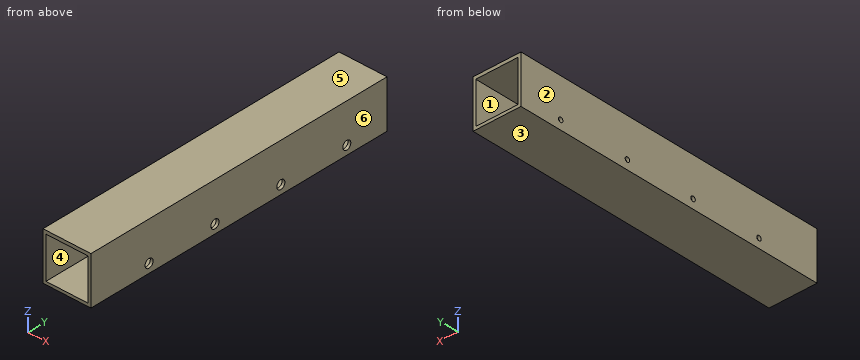
```python
from build123d import *

# Parameters (mm, degrees)
F0_W     = 50.8
F0_H     = 50.8
F0_W_2   = 44.7234460877
F0_H_2   = 44.0774458626
F1_DEPTH = 168.275
F3_D     = 9.144
F3_DEPTH = 25.4
F3_TIP   = 2.7471347502
F5_D     = 5.08
F5_DEPTH = 25.4
F5_TIP   = 1.5261859723


with BuildPart() as f1:
    # F0 (on Front) → F1 (new body, symmetric)
    with BuildSketch(Plane.XZ):
        with Locations((0.9841322899, 3.6690509832)):
            Rectangle(F0_W, F0_H)
        with Locations((1.1056640122, 3.467582593)):
            Rectangle(F0_W_2, F0_H_2, mode=Mode.SUBTRACT)
    extrude(amount=F1_DEPTH, both=True)

    # F3
    with Locations(Plane.YZ.offset(26.3841322899)):
        with Locations((-102.235, -12.3329490168), (-27.305, -12.3329490168), (47.625, -12.3329490168), (122.555, -12.3329490168)):
            Hole(F3_D / 2, depth=F3_DEPTH)
            with Locations((0, 0, -(F3_DEPTH + F3_TIP / 2))):  # 118° drill point
                Cone(0, F3_D / 2, F3_TIP, mode=Mode.SUBTRACT)

    # F5
    with Locations(Plane(origin=(-24.4158677101, 0, 0), x_dir=(0, -1, 0), z_dir=(-1, 0, 0))):
        with Locations((-123.0434924364, -12.0630878955), (-47.2589172423, -12.0630878955), (27.3903068155, -12.0630878955), (102.3233607411, -12.0630878955)):
            Hole(F5_D / 2, depth=F5_DEPTH)
            with Locations((0, 0, -(F5_DEPTH + F5_TIP / 2))):  # 118° drill point
                Cone(0, F5_D / 2, F5_TIP, mode=Mode.SUBTRACT)


solid = f1.part
```
Build history of the part. All positions in model axes, mm. Face numbers are marked on the shaded views. A direction names the side the tool comes from. Round coordinates to 2 decimals unless told otherwise and drop trailing zeros. Write each loop counter-clockwise with the first axis right and the second up, starting at its lowest first coordinate (ties: lowest second). Pieces come first, ordered by that corner, then holes.
1) Band-saw the part on B-B, the plane x = 6.5. List the corners of the cut face in (y, z) (3 decimals), and give its area (3 significant figures).
2) 3-axis set-ups, long thin cutter, end or side, ignore diameter. For the marked faces 1 and 2: which of +Z, -Z, +X, -X, +Y, -Y reach the whole face in a straight line?
3) Band-saw the part on C-C, the plane y = 6.5. List the corners of the cut face in (x, z).
4) Drill centre lines: probe 1 along Z at (x, y) = (-11.5, 6.5); probe 2 along X at (y, z) = (113, -2.5). Where is each one in solid material? Low to high.
5) Mould opens along Z. For the marked faces 3, 4, 5 and 6 say: +Z half, -Z half, draft (parallel to the pull), parting line (faces both ways), or undercut.
6) Pin check, flat tips, straight feed: pin 1 (4 mm diameter, centred on y = -102.32, z = -12.06, fed in from +X); pin 2 (7.5 mm diameter, centred on y = -27.3, z = -12.33, fed in from +X). Stop position of each tip, or through.
7) Band-saw the part on A-A, the plane z = 3. List the corners of the cut face in (x, y) (3 decimals), and give its area (3 significant figures).
Ans:
1. outline: (-168.275, -21.731) - (168.275, -21.731) - (168.275, -18.571) - (-168.275, -18.571) - close; (-168.275, 25.506) - (168.275, 25.506) - (168.275, 29.069) - (-168.275, 29.069) - close
1. area: 2,260 mm2
2. face 1: +Y, -Y
2. face 2: +Z, -Z, -X, +Y, -Y
3. outline: (-24.42, -21.73) - (26.38, -21.73) - (26.38, 29.07) - (-24.42, 29.07) - close; hole (-21.26, -18.57) - (23.47, -18.57) - (23.47, 25.51) - (-21.26, 25.51) - close
4. probe 1: z = -21.73 to -18.57, 25.51 to 29.07
4. probe 2: x = -24.42 to -21.26, 23.47 to 26.38
5. face 3: -Z half
5. face 4: undercut
5. face 5: +Z half
5. face 6: draft
6. pin 1: passes through
6. pin 2: stops at x = -21.26
7. outline: (-24.416, -168.275) - (-21.256, -168.275) - (-21.256, 168.275) - (-24.416, 168.275) - close; (23.467, -168.275) - (26.384, -168.275) - (26.384, 168.275) - (23.467, 168.275) - close
7. area: 2,050 mm2
